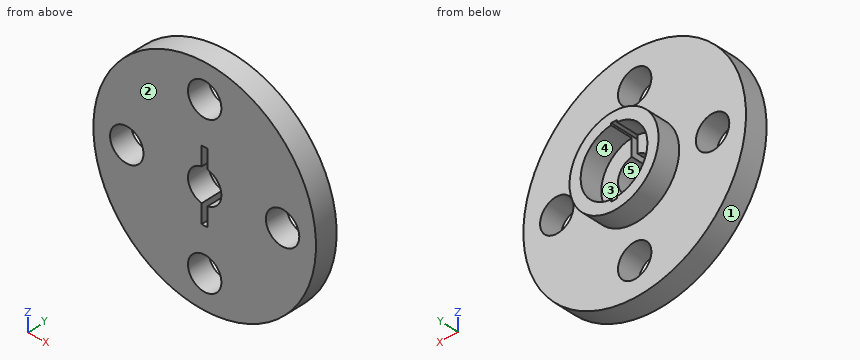
from build123d import *

# Parameters (mm, degrees)
SKETCH_1_R          = 10
SKETCH_1_R_2        = 1.5
EXTRUDE_1_DEPTH     = 2
SKETCH_2_R          = 4
SKETCH_2_R_2        = 3
EXTRUDE_2_DEPTH     = 2
SKETCH_3_W          = 0.526425496
SKETCH_3_H          = 6.332921184
CUT_EXTRUDE_1_DEPTH = 4


with BuildPart() as part:
    # 草图1 → 凸台-拉伸1 (new body)
    with BuildSketch(Plane(origin=(0, 0, 0), x_dir=(1, 0, 0), z_dir=(0, 1, 0))):
        with Locations(Location((0, 0, 0), (0, 0, 270))):
            Circle(SKETCH_1_R)
        with Locations(Location((7, 0, 0), (0, 0, 270))):
            Circle(SKETCH_1_R_2, mode=Mode.SUBTRACT)
        with Locations(Location((0, 0, 0), (0, 0, 270))):
            Circle(SKETCH_1_R_2, mode=Mode.SUBTRACT)
        with Locations(Location((0, -7, 0), (0, 0, 270))):
            Circle(SKETCH_1_R_2, mode=Mode.SUBTRACT)
        with Locations(Location((-7, 0, 0), (0, 0, 270))):
            Circle(SKETCH_1_R_2, mode=Mode.SUBTRACT)
        with Locations(Location((0, 7, 0), (0, 0, 270))):
            Circle(SKETCH_1_R_2, mode=Mode.SUBTRACT)
    extrude(amount=EXTRUDE_1_DEPTH)

    # 草图2 → 凸台-拉伸2 (add)
    with BuildSketch(Plane(origin=(0, 2, 0), x_dir=(1, 0, 0), z_dir=(0, 1, 0))):
        with Locations(Location((0, 0, 0), (0, 0, 270))):
            Circle(SKETCH_2_R)
        with Locations(Location((0, 0, 0), (0, 0, 270))):
            Circle(SKETCH_2_R_2, mode=Mode.SUBTRACT)
    extrude(amount=EXTRUDE_2_DEPTH)

    # 草图3 → 切除-拉伸1 (cut)
    with BuildSketch(Plane.XZ):
        Rectangle(SKETCH_3_W, SKETCH_3_H)
    extrude(amount=-CUT_EXTRUDE_1_DEPTH, mode=Mode.SUBTRACT)


solid = part.part
For this review, take the finished solid that the model builds, in its own axes (mm). Face numbers are marked on the shaded views. A direction names the side the tool comes from. Coordinates: 2 decimals unless noted, no trailing zeros. Loops run counter-clockwise (first coordinate to the right, second up) from the corner with the lowest first, then second, coordinate; pieces in that order, holes last. Notation, with made-up numbers: (56, 1.25) -> (71, 1.25) arc R17 ccw to (71, 20.25) -> close; hole circle Ø1 at (-24, 29). An arc over 180 degrees is marked (long way). Write each question's results on one line, items separated by ' | '.
Q1. Add section C-C, the plane y = 3.35. State the section outline as (x, z) points, then the cut area to 3 significant figures.
Taken from the geometry:
outline: circle Ø8 at (0, 0); hole (-0.26, -3.17) -> (0.26, -3.17) -> (0.26, -2.99) arc R3 ccw to (0.26, 2.99) -> (0.26, 3.17) -> (-0.26, 3.17) -> (-0.26, 2.99) arc R3 ccw to (-0.26, -2.99) -> close | area: 21.8 mm²
Q2. Add section A-A, the plane y = 1.2. State the section outline as (x, z) points.
Taken from the geometry:
outline: circle Ø20 at (0, 0); hole circle Ø3 at (-7, 0); hole circle Ø3 at (0, -7); hole circle Ø3 at (0, 7); hole (-0.26, -3.17) -> (0.26, -3.17) -> (0.26, -1.48) arc R1.5 ccw to (0.26, 1.48) -> (0.26, 3.17) -> (-0.26, 3.17) -> (-0.26, 1.48) arc R1.5 ccw to (-0.26, -1.48) -> close; hole circle Ø3 at (7, 0)
Q3. Machinability: for the marked faces 4 and 5, which of the approach directions +Z, -Z, +X, -X, +Y, -Y give a long, thin tool a straight path to every point of the face, cutting with its end or side? Answer none if there is none.
Taken from the geometry:
face 4: +Y | face 5: +Y, -Y
Q4. For pin 1 Ø2 at (x, z) = (1.5, 0.5) entering from +Y; pin 2 Ø1.5 at (y, z) = (1, -6.5) entering from +X; pin 3 Ø0.5 at (y, z) = (1.5, -2.5) entering from +X, all flat-tipped, find the tip position at first contact; note any pin that passes through.
Taken from the geometry:
pin 1: y = 2 | pin 2: x = 8.18 | pin 3: x = 9.74
Q5. To check wall thickness, follow line 1 along X through (y, z) = (1.65, 0); line 2 along Y through (x, z) = (-4, 0.5); line 3 along Z through (x, y) = (-2.75, 3.1). State the ranges of each line that lie inside material, in increasing order. Write a range as [from, to].
Taken from the geometry:
line 1: [-10, -8.5], [-5.5, -1.5], [1.5, 5.5], [8.5, 10] | line 2: [0, 2] | line 3: [-2.9, -1.2], [1.2, 2.9]
Q6. Add section B-B, the plane z = 6. State the section outline as (x, y) points.
Taken from the geometry:
outline: (-8, 0) -> (-1.12, 0) -> (-1.12, 2) -> (-8, 2) -> close; (1.12, 0) -> (8, 0) -> (8, 2) -> (1.12, 2) -> close
Q7. Add section D-D, the plane z = 0.5. State the section outline as (x, y) points.
Taken from the geometry:
outline: (-9.99, 0) -> (-8.41, 0) -> (-8.41, 2) -> (-9.99, 2) -> close; (-5.59, 0) -> (-1.41, 0) -> (-1.41, 2) -> (-2.96, 2) -> (-2.96, 4) -> (-3.97, 4) -> (-3.97, 2) -> (-5.59, 2) -> close; (1.41, 0) -> (5.59, 0) -> (5.59, 2) -> (3.97, 2) -> (3.97, 4) -> (2.96, 4) -> (2.96, 2) -> (1.41, 2) -> close; (8.41, 0) -> (9.99, 0) -> (9.99, 2) -> (8.41, 2) -> close
Q8. Mouldability with a two-part tool opening along X and no side actions: class the marked faces 1, 2 and 3 as +X half, -X half, draft (parallel to the pull), parting line (faces both ways), or undercut.
Taken from the geometry:
face 1: parting line | face 2: draft | face 3: undercut
